Could you check a few things on this model? Use its own coordinates, in mm. Face numbers are marked on the shaded views. A direction names the side the tool comes from. Give positions to 0.01 mm unless a question says otherwise; leave off trailing zeros. Order: outer loops, then holes, each group sorted by start corner. A loop starts at its lowest first (then second) coordinate and runs counter-clockwise, first axis right, second up. Notation, with made-up numbers: M 42,79 L 55,79 A18 ccw 55,101 Z; hole C -24,54.25 d1. An arc over 180 degrees is marked long. Answer in a Markdown table with one row per item. Add a question column.
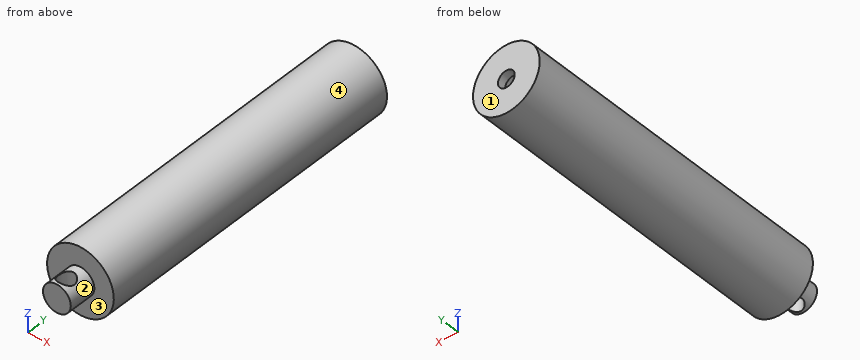
```python
from build123d import *

# Parameters (mm, degrees)
CUT_EXTRUDE_1_DEPTH      = 128.137720603
CUT_EXTRUDE_1_DEPTH_BACK = 128.137720603
SKETCH_2_R               = 3


with BuildPart() as part:
    # 草图1 → 旋转1 (revolve)
    with BuildSketch(Plane.XY, mode=Mode.PRIVATE) as revolve_1_sk:
        Polygon((0, 0), (-5, 0), (-5, 10), (-12, 10), (-12, 126), (-3, 126), (-3, 123), (-10, 123), (-10, 13), (0, 13), align=None)
    revolve(revolve_1_sk.sketch.rotate(Axis((0, 0, 0), (0, 1, 0)), 270), axis=Axis((0, 0, 0), (0, 1, 0)))

    # 草图2 → 切除-拉伸1 (cut, two sides: drawn at the far end of the back side and taken through both)
    with BuildSketch(Plane.XY.offset(-CUT_EXTRUDE_1_DEPTH_BACK)):
        with Locations((0, 3.963259356)):
            Circle(SKETCH_2_R)
    extrude(amount=CUT_EXTRUDE_1_DEPTH + CUT_EXTRUDE_1_DEPTH_BACK, mode=Mode.SUBTRACT)


solid = part.part
```
1. Suppose I cut it at C-C on y = 73. List the corners of the cut face in (x, z) for me.
2. Suppose I cut it at A-A on x = 0. List the corners of the cut face in (y, z) for me.
3. Suppose I cut it at D-D on x = 7.75. List the corners of the cut face in (y, z) for me.
4. Suppose I cut it at B-B on z = -7.5. List the corners of the cut face in (x, y) for me.
5. If I drill on line 1 along Y through (x, z) = (-4.25, -5); line 2 along X through (y, z) = (50.5, 0); line 3 along Y through (x, z) = (0, -1.25), over which ranges is the centre line in solid material (lowest first)? Write a range as [from, to].
6. Will these pins go through, and if not, where does the flat tip stop? P1, Ø1, axis at x = -6.5, y = 72, coming from the +Z side; P2, Ø1, axis at x = -9, y = 87.5, coming from the +Z side; P3, Ø1.5, axis at x = 6.5, y = 24, coming from the -Z side; P4, Ø5, axis at x = 0, y = 3.96, coming from the +Z side.
7. Thinking about a two-plate mould opening in Z: for the marked faces 3 and 4, which applies, pulls with the +Z half, pulls with the -Z half, needs draft (parallel to the pull), parting line crosses it, or undercut?
8. For the marked faces 1 and 2, which set-ups out of +Z, -Z, +X, -X, +Y, -Y let a thin tool reach every point of the face, with its end or its side?
Findings below:
| question | item | result |
|---|---|---|
| 1 | outline | C 0,0 d24; hole C 0,0 d20 |
| 2 | outline | M 0,-5 L 0.96,-5 L 0.96,5 L 0,5 Z; M 6.96,-5 L 10,-5 L 10,-12 L 126,-12 L 126,-3 L 123,-3 L 123,-10 L 13,-10 L 13,10 L 123,10 L 123,3 L 126,3 L 126,12 L 10,12 L 10,5 L 6.96,5 Z |
| 3 | outline | M 10,-9.16 L 126,-9.16 L 126,9.16 L 10,9.16 Z; hole M 13,-6.32 L 123,-6.32 L 123,6.32 L 13,6.32 Z |
| 4 | outline | M -9.37,10 L 9.37,10 L 9.37,126 L -9.37,126 Z; hole M -6.61,13 L 6.61,13 L 6.61,123 L -6.61,123 Z |
| 5 | line 1 | [10, 13], [123, 126] |
| 5 | line 2 | [-12, -10], [10, 12] |
| 5 | line 3 | [0, 0.96], [6.96, 13] |
| 6 | P1 | z = 10.39 |
| 6 | P2 | z = 8.47 |
| 6 | P3 | z = -10.53 |
| 6 | P4 | through |
| 7 | face 3 | needs draft |
| 7 | face 4 | parting line crosses it |
| 8 | face 1 | +Z, -Z, +X, -X, +Y |
| 8 | face 2 | -Y |
